The model under review builds one solid part; all positions refer to its coordinate system, in mm. Face numbers are marked on the shaded views. A direction names the side the tool comes from. Round coordinates to 2 decimals unless told otherwise and drop trailing zeros. Write each loop counter-clockwise with the first axis right and the second up, starting at its lowest first coordinate (ties: lowest second). Pieces come first, ordered by that corner, then holes.
Item 1: Add section A-A (z = 3). Give the boundary of the cut face in (x, y).
Item 2: To check wall thickness, follow L1, parallel to Y at x = 4, z = 3.5; L2, parallel to Y at x = 15.5, z = 5; L3, parallel to Z at x = 16, y = -0.9. State the ranges of each line that lie inside material, in increasing order.
Item 3: Add section C-C (x = 4). Give the boundary of the cut face in (y, z), plus the area to 3 significant figures.
Item 4: Draft analysis for pull direction Y (two halves, no side actions). For the marked faces 1, 2 and 3, state which applies: +Y half, -Y half, draft (parallel to the pull), parting line (faces both ways), or undercut.
Item 5: Machinability: for the marked faces 4 and 5, which of the approach directions +Z, -Z, +X, -X, +Y, -Y give a long, thin tool a straight path to every point of the face, cutting with its end or side? Answer none if there is none.
Item 6: Clearance check with a flat-ended pin moving along its axis: pin 1 Ø3 at (x, y) = (4, 3.5) entering from -Z. State where the tip first meets the part, or that it passes through.
Item 7: Add section B-B (y = 3.5). Give the boundary of the cut face in (x, z).
Item 8: Add section D-D (x = 16). Give the boundary of the cut face in (y, z), plus the area to 3 significant figures.
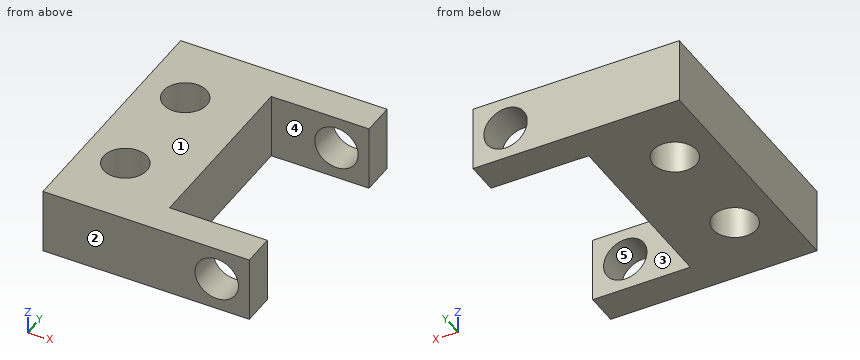
```python
from build123d import *

# Parameters (mm, degrees)
CYLINDER003_R          = 2
CYLINDER003_DEPTH      = 25
CYLINDER003_ROLL_ANGLE = 90
BOX001_W               = 19
BOX001_H               = 3
BOX001_DEPTH           = 6
BOX002_W               = 19
BOX002_H               = 3
BOX002_DEPTH           = 6
CYLINDER002_R          = 2
CYLINDER002_DEPTH      = 10
CYLINDER001_R          = 2
CYLINDER001_DEPTH      = 10
CYLINDER_R             = 2
CYLINDER_DEPTH         = 10
BOX_W                  = 10
BOX_H                  = 17
BOX_DEPTH              = 6


with BuildPart() as cylinder003:
    # Cylinder003 → Cylinder003 (new body)
    with BuildSketch(Plane.XY):
        Circle(CYLINDER003_R)
    extrude(amount=CYLINDER003_DEPTH)


with BuildPart() as cylinder003_1:
    # Cylinder003 roll: moved
    add(cylinder003.part.rotate(Axis((0, 0, 0), (1, 0, 0)), CYLINDER003_ROLL_ANGLE))


with BuildPart() as cylinder003_2:
    # Cylinder003 placement: moved
    add(cylinder003_1.part.moved(Location((16, 21, 3))))


with BuildPart() as cube001:
    # Box001 → Box001 (new body)
    with BuildSketch(Plane(origin=(0, -3, 0), x_dir=(1, 0, 0), z_dir=(0, 0, 1))):
        with Locations((9.5, 1.5)):
            Rectangle(BOX001_W, BOX001_H)
    extrude(amount=BOX001_DEPTH)


with BuildPart() as cube002:
    # Box002 → Box002 (new body)
    with BuildSketch(Plane(origin=(0, 17, 0), x_dir=(1, 0, 0), z_dir=(0, 0, 1))):
        with Locations((9.5, 1.5)):
            Rectangle(BOX002_W, BOX002_H)
    extrude(amount=BOX002_DEPTH)


with BuildPart() as cylinder002:
    # Cylinder002 → Cylinder002 (new body)
    with BuildSketch(Plane(origin=(4, 13.5, 0), x_dir=(1, 0, 0), z_dir=(0, 0, 1))):
        Circle(CYLINDER002_R)
    extrude(amount=CYLINDER002_DEPTH)


with BuildPart() as cylinder001:
    # Cylinder001 → Cylinder001 (new body)
    with BuildSketch(Plane(origin=(4, 3.5, 0), x_dir=(1, 0, 0), z_dir=(0, 0, 1))):
        Circle(CYLINDER001_R)
    extrude(amount=CYLINDER001_DEPTH)


with BuildPart() as cylinder:
    # Cylinder → Cylinder (new body)
    with BuildSketch(Plane(origin=(4, 3.5, 0), x_dir=(1, 0, 0), z_dir=(0, 0, 1))):
        Circle(CYLINDER_R)
    extrude(amount=CYLINDER_DEPTH)


with BuildPart() as cut003:
    # Box → Box (new body)
    with BuildSketch(Plane.XY):
        with Locations((5, 8.5)):
            Rectangle(BOX_W, BOX_H)
    extrude(amount=BOX_DEPTH)

    # Cut: cut Cylinder
    add(cylinder.part, mode=Mode.SUBTRACT)

    # Cut001: cut Cylinder001
    add(cylinder001.part, mode=Mode.SUBTRACT)

    # Cut002: cut Cylinder002
    add(cylinder002.part, mode=Mode.SUBTRACT)

    # Fusion: union Cube001, Cube002
    add(cube001.part)
    add(cube002.part)

    # Cut003: cut Cylinder003
    add(cylinder003_2.part, mode=Mode.SUBTRACT)


solid = cut003.part
```
Numbers:
1. outline: (0, -3) - (14, -3) - (14, 0) - (10, 0) - (10, 17) - (14, 17) - (14, 20) - (0, 20) - close; (18, -3) - (19, -3) - (19, 0) - (18, 0) - close; (18, 17) - (19, 17) - (19, 20) - (18, 20) - close; hole circle Ø4 at (4, 3.5); hole circle Ø4 at (4, 13.5)
2. L1: y = -3 to 1.5, 5.5 to 11.5, 15.5 to 20
2. L2: y = -3 to 0, 17 to 20
2. L3: z = 0 to 1, 5 to 6
3. outline: (-3, 0) - (1.5, 0) - (1.5, 6) - (-3, 6) - close; (5.5, 0) - (11.5, 0) - (11.5, 6) - (5.5, 6) - close; (15.5, 0) - (20, 0) - (20, 6) - (15.5, 6) - close
3. area: 90.0 mm2
4. face 1: draft
4. face 2: -Y half
4. face 3: undercut
5. face 4: +Z, -Z, +X
5. face 5: +Y, -Y
6. pin 1: passes through
7. outline: (0, 0) - (2, 0) - (2, 6) - (0, 6) - close; (6, 0) - (10, 0) - (10, 6) - (6, 6) - close
8. outline: (-3, 0) - (0, 0) - (0, 1) - (-3, 1) - close; (-3, 5) - (0, 5) - (0, 6) - (-3, 6) - close; (17, 0) - (20, 0) - (20, 1) - (17, 1) - close; (17, 5) - (20, 5) - (20, 6) - (17, 6) - close
8. area: 12.0 mm2
